```python
from build123d import *

# Parameters (mm, degrees)
SKETCH1_W           = 60
SKETCH1_H           = 90
BOSS_EXTRUDE1_DEPTH = 15
SKETCH2_R           = 30
BOSS_EXTRUDE2_DEPTH = 30
SKETCH3_R           = 8
BOSS_EXTRUDE3_DEPTH = 15


with BuildPart() as part:
    # Sketch1 → Boss-Extrude1 (new body)
    with BuildSketch(Plane.XY):
        Rectangle(SKETCH1_W, SKETCH1_H)
    extrude(amount=BOSS_EXTRUDE1_DEPTH)

    # Sketch2 → Boss-Extrude2 (add)
    with BuildSketch(Plane.XY.offset(15)):
        Circle(SKETCH2_R)
        with BuildLine():
            Line((-4.058122732, -14.440624637), (-4.058122732, -17.999887391))
            Line((-4.058122732, -17.999887391), (3.941877268, -17.999887391))
            Line((3.941877268, -17.999887391), (3.941877268, -14.472788384))
            ThreePointArc((3.941877268, -14.472788384), (0.060306539, 14.99987877), (-4.058122732, -14.440624637))
        make_face(mode=Mode.SUBTRACT)
    extrude(amount=BOSS_EXTRUDE2_DEPTH)

    # Sketch3 → Boss-Extrude3 (add)
    with BuildSketch(Plane(origin=(0, 45, 0), x_dir=(1, 0, 0), z_dir=(0, 1, 0))):
        with BuildLine():
            Line((-30, 0), (30, 0))
            Line((30, 0), (22.03289839, 26.599347585))
            ThreePointArc((22.03289839, 26.599347585), (0, 43), (-22.03289839, 26.599347585))
            Line((-22.03289839, 26.599347585), (-30, 0))
        make_face()
        with Locations((0, 20)):
            Circle(SKETCH3_R, mode=Mode.SUBTRACT)
    boss_extrude3 = extrude(amount=-BOSS_EXTRUDE3_DEPTH)

    # Mirror1: Boss-Extrude3 across plane
    add(boss_extrude3.mirror(Plane.ZX))


solid = part.part
```
Can you work these out from the model? Positions are in its coordinate system, mm. A direction names the side the tool comes from. Coordinates: 2 decimals unless noted, no trailing zeros. Loops run counter-clockwise (first coordinate to the right, second up) from the corner with the lowest first, then second, coordinate; pieces in that order, holes last. Notation, with made-up numbers: (74.5, 3) -> (78.5, 3) arc R15 ccw to (78.5, 22) -> close; hole circle Ø8 at (65.25, 29). An arc over 180 degrees is marked (long way). Put each result on its own line as item: value. Start each with the question number.
Q1. I want a section at A-A (x = 0). Write out the boundary of the cut face in (y, z).
Q2. For faces 5 (the face through (0, -32, 15)), 6 (the face through (6, 30, -12)), 7 (the face through (0, -18, 30)), 8 (the face through (0, 38, -43)), which set-ups out of +Z, -Z, +X, -X, +Y, -Y let a thin tool reach every point of the face, with its end or its side?
Q3. If I drill on line 1 (Y direction, x = 0, z = 34); line 2 (Y direction, x = 11, z = -35.5); line 3 (X direction, y = -35, z = -27), over which ranges is the centre line in solid material (lowest first)? Write a range as [from, to].
Q4. I want a section at D-D (z = 34). Write out the boundary of the cut face in (x, y), plus the area to 3 significant figures.
Q5. Thinking about a two-plate mould opening in X: for faces 1 (the face through (6, 14, 45)), 2 (the face through (-1.041, 37.605, -27.932)), 3 (the face through (-29.97, 1.32, 29.79)), 4 (the face through (-25.96, -37.61, -13.49)), which applies, pulls with the +X half, pulls with the -X half, needs draft (parallel to the pull), parting line crosses it, or undercut?
Q6. I'm going to push flat-ended pins straight in: P1, Ø10, axis at x = -1, y = 3, coming from the +Z side; P2, Ø1.5, axis at y = -26, z = 29.5, coming from the +X side; P3, Ø5, axis at x = 19.5, y = -16, coming from the -Z side. Where does each tip first touch, or does it pass through?
Q7. I want a section at B-B (y = 33). Write out the boundary of the cut face in (x, z), plus the area to 3 significant figures.
Q8. I want a section at C-C (z = -20). Write out the boundary of the cut face in (x, y), plus the area to 3 significant figures.
Taken from the geometry:
1. outline: (-45, -43) -> (-30, -43) -> (-30, -28) -> (-45, -28) -> close; (-45, -12) -> (-30, -12) -> (-30, 0) -> (30, 0) -> (30, -12) -> (45, -12) -> (45, 15) -> (30, 15) -> (30, 45) -> (15, 45) -> (15, 15) -> (-18, 15) -> (-18, 45) -> (-30, 45) -> (-30, 15) -> (-45, 15) -> close; (30, -43) -> (45, -43) -> (45, -28) -> (30, -28) -> close
2. face 5: +Z, -Y
2. face 6: -Z, +X, -X
2. face 7: +Z
2. face 8: -Z, +Y, -Y
3. line 1: y = [-30, -18], [15, 30]
3. line 2: y = [-45, -30], [30, 45]
3. line 3: x = [-21.91, -3.87], [3.87, 21.91]
4. outline: circle Ø60 at (0, 0); hole (-4.06, -18) -> (3.94, -18) -> (3.94, -14.47) arc R15 ccw (long way) to (-4.06, -14.44) -> close
4. area: 2,100 mm2
5. face 1: needs draft
5. face 2: undercut
5. face 3: parting line crosses it
5. face 4: pulls with the -X half
6. P1: stops at z = 15
6. P2: stops at x = 16.2
6. P3: stops at z = 0
7. outline: (-30, 0) -> (-22.03, -26.6) arc R23 ccw to (22.03, -26.6) -> (30, 0) -> (30, 15) -> (-30, 15) -> close; hole circle Ø16 at (0, -20)
7. area: 2,610 mm2
8. outline: (-24.01, -45) -> (-8, -45) -> (-8, -30) -> (-24.01, -30) -> close; (-24.01, 30) -> (-8, 30) -> (-8, 45) -> (-24.01, 45) -> close; (8, -45) -> (24.01, -45) -> (24.01, -30) -> (8, -30) -> close; (8, 30) -> (24.01, 30) -> (24.01, 45) -> (8, 45) -> close
8. area: 961 mm2
